```python
from build123d import *

# Parameters (mm, degrees)
BOSS_EXTRUDE1_DEPTH                = 9
BOSS_EXTRUDE2_DEPTH                = 15.4
BOSS_EXTRUDE3_DEPTH                = 9
SKETCH4_R                          = 4.5
CUT_EXTRUDE1_DEPTH                 = 5
SKETCH5_R                          = 2.5
BOSS_EXTRUDE4_DEPTH                = 26.9
SKETCH6_W                          = 16.2
SKETCH6_H                          = 1.547449217
BOSS_EXTRUDE5_DEPTH                = 3.5
EXTRUDE_THIN4_DEPTH                = 6
BOSS_EXTRUDE7_DEPTH                = 0.5
SKETCH9_W                          = 16.123667198
SKETCH9_H                          = 0.274090176
BOSS_EXTRUDE8_DEPTH                = 3.5
SKETCH10_R                         = 0.25
BOSS_EXTRUDE9_DEPTH                = 5.5
CHAMFER1_SIZE                      = 0.1
SKETCH11_R                         = 11
SKETCH11_R_2                       = 4.5
BOSS_EXTRUDE10_DEPTH               = 2.5
FILLET1_R                          = 1
CUT_EXTRUDE2_DEPTH                 = 18
FILLET2_R                          = 0.5
TAP_DRILL_FOR_M2_5X0_45_TAP2_D     = 2.05
TAP_DRILL_FOR_M2_5X0_45_TAP2_DEPTH = 5
TAP_DRILL_FOR_M2_5X0_45_TAP2_TIP   = 0.615882135


with BuildPart() as part:
    # Sketch1 → Boss-Extrude1 (new body)
    with BuildSketch(Plane.XY):
        Polygon((21, 16.5), (16.5, 21), (-16.5, 21), (-21, 16.5), (-21, -16.5), (-16.5, -21), (16.5, -21), (21, -16.5), align=None)
    extrude(amount=BOSS_EXTRUDE1_DEPTH)

    # Sketch2 → Boss-Extrude2 (add)
    with BuildSketch(Plane.XY.offset(9)):
        with BuildLine():
            Line((11, 20.9), (-11, 20.9))
            ThreePointArc((-11, 20.9), (-18.000357134, 18.000357134), (-20.9, 11))
            Line((-20.9, 11), (-20.9, -11))
            ThreePointArc((-20.9, -11), (-18.000357134, -18.000357134), (-11, -20.9))
            Line((-11, -20.9), (11, -20.9))
            ThreePointArc((11, -20.9), (18.000357134, -18.000357134), (20.9, -11))
            Line((20.9, -11), (20.9, 11))
            ThreePointArc((20.9, 11), (18.000357134, 18.000357134), (11, 20.9))
        make_face()
    extrude(amount=BOSS_EXTRUDE2_DEPTH)

    # Sketch3 → Boss-Extrude3 (add)
    with BuildSketch(Plane.XY.offset(24.4)):
        Polygon((21, -16.5), (21, 16.5), (16.5, 21), (-16.5, 21), (-21, 16.5), (-21, -16.5), (-16.5, -21), (16.5, -21), align=None)
    extrude(amount=BOSS_EXTRUDE3_DEPTH)

    # Sketch4 → Cut-Extrude1 (cut)
    with BuildSketch(Plane.XY.offset(33.4)):
        Circle(SKETCH4_R)
    extrude(amount=-CUT_EXTRUDE1_DEPTH, mode=Mode.SUBTRACT)

    # Sketch5 → Boss-Extrude4 (add)
    with BuildSketch(Plane.XY.offset(28.4)):
        Circle(SKETCH5_R)
    extrude(amount=BOSS_EXTRUDE4_DEPTH)

    # Sketch6 → Boss-Extrude5 (add)
    with BuildSketch(Plane(origin=(0, 21, 0), x_dir=(1, 0, 0), z_dir=(0, 1, 0))):
        with Locations((0, -0.773724609)):
            Rectangle(SKETCH6_W, SKETCH6_H)
    extrude(amount=BOSS_EXTRUDE5_DEPTH)

    # Sketch7 → Extrude-Thin4 (add)
    with BuildSketch(Plane(origin=(0, 21, 0), x_dir=(1, 0, 0), z_dir=(0, 1, 0))):
        Polygon((-5.1, -8.547449217), (-8.1, -8.547449217), (-8.1, -2.547449217), (8.1, -2.547449217), (8.1, -8.547449217), (5.1, -8.547449217), (5.1, -8.047449217), (7.6, -8.047449217), (7.6, -3.047449217), (-7.6, -3.047449217), (-7.6, -8.047449217), (-5.1, -8.047449217), align=None)
    extrude(amount=EXTRUDE_THIN4_DEPTH)

    # Sketch8 → Boss-Extrude7 (add)
    with BuildSketch(Plane(origin=(0, 21, 0), x_dir=(1, 0, 0), z_dir=(0, 1, 0))):
        Polygon((-5.1, -8.047449217), (-5.1, -8.547449217), (5.1, -8.547449217), (5.1, -8.047449217), (7.6, -8.047449217), (7.6, -3.047449217), (-7.6, -3.047449217), (-7.6, -8.047449217), align=None)
    extrude(amount=BOSS_EXTRUDE7_DEPTH)

    # Sketch9 → Boss-Extrude8 (add)
    with BuildSketch(Plane(origin=(0, 21, 0), x_dir=(1, 0, 0), z_dir=(0, 1, 0))):
        with Locations((0, -2.039705449)):
            Rectangle(SKETCH9_W, SKETCH9_H)
    extrude(amount=BOSS_EXTRUDE8_DEPTH)

    # Sketch10 → Boss-Extrude9 (add)
    with BuildSketch(Plane(origin=(0, 21.5, 0), x_dir=(1, 0, 0), z_dir=(0, 1, 0))):
        with Locations((-6.204552759, -5.547449217)):
            Circle(SKETCH10_R)
        with Locations((-3.704552759, -5.547449217)):
            Circle(SKETCH10_R)
        with Locations((-1.204552759, -5.547449217)):
            Circle(SKETCH10_R)
        with Locations((1.295447241, -5.547449217)):
            Circle(SKETCH10_R)
        with Locations((3.795447241, -5.547449217)):
            Circle(SKETCH10_R)
        with Locations((6.295447241, -5.547449217)):
            Circle(SKETCH10_R)
    extrude(amount=BOSS_EXTRUDE9_DEPTH)

    # Chamfer1
    chamfer1_edges = [part.edges().sort_by_distance(p)[0] for p in [
        (-6.454552759, 27, 5.547449217),
        (-3.954552759, 27, 5.547449217),
        (-1.454552759, 27, 5.547449217),
        (1.045447241, 27, 5.547449217),
        (3.545447241, 27, 5.547449217),
        (6.045447241, 27, 5.547449217),
    ]]
    chamfer(chamfer1_edges, length=CHAMFER1_SIZE)

    # Sketch11 → Boss-Extrude10 (add)
    with BuildSketch(Plane.XY.offset(33.4)):
        Circle(SKETCH11_R)
        Circle(SKETCH11_R_2, mode=Mode.SUBTRACT)
    extrude(amount=BOSS_EXTRUDE10_DEPTH)

    # Fillet1
    fillet1_edges = [part.edges().sort_by_distance(p)[0] for p in [
        (-11, 0, 33.4),
    ]]
    fillet(fillet1_edges, radius=FILLET1_R)

    # Sketch12 → Cut-Extrude2 (cut)
    with BuildSketch(Plane.XY.offset(55.3)):
        with BuildLine():
            Line((2, 1.5), (-2, 1.5))
            ThreePointArc((-2, 1.5), (0, 2.5), (2, 1.5))
        make_face()
    extrude(amount=-CUT_EXTRUDE2_DEPTH, mode=Mode.SUBTRACT)

    # Fillet2
    fillet2_edges = [part.edges().sort_by_distance(p)[0] for p in [
        (-0.790569415, -2.371708245, 55.3),
    ]]
    fillet(fillet2_edges, radius=FILLET2_R)

    # Tap Drill for M2.5x0.45 Tap2
    with Locations(Plane.XY.offset(33.4)):
        with Locations((15.5, 16.5), (15.5, -16.5), (-15.5, -16.5), (-15.5, 16.5)):
            Hole(TAP_DRILL_FOR_M2_5X0_45_TAP2_D / 2, depth=TAP_DRILL_FOR_M2_5X0_45_TAP2_DEPTH)
            with Locations((0, 0, -(TAP_DRILL_FOR_M2_5X0_45_TAP2_DEPTH + TAP_DRILL_FOR_M2_5X0_45_TAP2_TIP / 2))):  # 118° drill point
                Cone(0, TAP_DRILL_FOR_M2_5X0_45_TAP2_D / 2, TAP_DRILL_FOR_M2_5X0_45_TAP2_TIP, mode=Mode.SUBTRACT)


solid = part.part
```
Geometry: final body of the model. Coordinates: model frame, mm. A direction names the side the tool comes from. Give positions to 0.01 mm unless a question says otherwise; leave off trailing zeros. Order: outer loops, then holes, each group sorted by start corner. A loop starts at its lowest first (then second) coordinate and runs counter-clockwise, first axis right, second up. Notation, with made-up numbers: M 81.25,25 L 130.25,25 A29 cw 130.25,64 Z; hole C 64,78 d2. An arc over 180 degrees is marked long. Answer as CSV lines item,"result". Start each with the question number.
1) First-contact query: P1, Ø7.5, axis at x = -3, z = 14, coming from the -Y side; P2, Ø6.5, axis at x = 0.5, y = 25.5, coming from the +Z side; P3, Ø2.5, axis at y = 24, z = 5.5, coming from the +X side. Flat tips, straight axial feed; report the tip coordinate or a pass-through.
2) Mould query, pull axis X, two halves, no side actions, for faces 1 (the flat face through (2, -2, 28.4)), 2 (the flat face through (8.1, 24, 6)), 3 (the flat face through (0, 23, 2.177)). Classes: +X half, -X half, draft (parallel to the pull), parting line (faces both ways), or undercut.
3) Line query: line 1 (Y direction, x = -15.5, z = 32.35) (3 decimals); line 2 (Y direction, x = 0, z = 30.5); line 3 (X direction, y = 16.5, z = 32) (3 decimals). Output: solid intervals per line, ascending. Write a range as from..to.
4) Cut plane C-C (x = -13). Output: boundary loops of the cut face in (y, z).
5) Cut plane B-B (z = 21.5). Output: boundary loops of the cut face in (x, y).
6) Cut plane D-D (z = 46.5). Output: boundary loops of the cut face in (x, y).
7) Cut plane A-A (y = 0). Output: boundary loops of the cut face in (x, z), then the cut area to 3 significant figures.
8) Set-up query: faces 4 (the flat face through (-8.1, 24, 6)), 5 (the flat face through (8.1, 23, 1)), 6 (the flat face through (7.6, 24, 6)), 7 (the cylindrical face through (15.633, 17.516, 30.865)). Return all of +Z, -Z, +X, -X, +Y, -Y with unobstructed straight access to the full face (end or side cutting, diameter ignored); none if empty.
Findings below:
1,P1,"stops at y = -20.9"
1,P2,"stops at z = 5.8"
1,P3,"stops at x = 8.1"
2,face 1,"undercut"
2,face 2,"+X half"
2,face 3,"draft"
3,line 1,"y = -21..-17.525, -15.475..15.475, 17.525..21"
3,line 2,"y = -21..-4.5, -2.5..2.5, 4.5..21"
3,line 3,"x = -21..-16.525, -14.475..14.475, 16.525..21"
4,outline,"M -21,0 L 21,0 L 21,9 L 20.7,9 L 20.7,24.4 L 21,24.4 L 21,33.4 L -21,33.4 L -21,24.4 L -20.7,24.4 L -20.7,9 L -21,9 Z"
5,outline,"M -20.9,-11 A9.9 ccw -11,-20.9 L 11,-20.9 A9.9 ccw 20.9,-11 L 20.9,11 A9.9 ccw 11,20.9 L -11,20.9 A9.9 ccw -20.9,11 Z"
6,outline,"M -2,1.5 A2.5 ccw long 2,1.5 Z"
7,outline,"M -21,0 L 21,0 L 21,9 L 20.9,9 L 20.9,24.4 L 21,24.4 L 21,33.4 L 12,33.4 A1 cw 11,34.4 L 11,35.9 L 4.5,35.9 L 4.5,28.4 L 2.5,28.4 L 2.5,54.8 A0.5 ccw 2,55.3 L -2,55.3 A0.5 ccw -2.5,54.8 L -2.5,28.4 L -4.5,28.4 L -4.5,35.9 L -11,35.9 L -11,34.4 A1 cw -12,33.4 L -21,33.4 L -21,24.4 L -20.9,24.4 L -20.9,9 L -21,9 Z"
7,area,"1,520 mm²"
8,face 4,"+Z, -Z, -X, +Y"
8,face 5,"+Z, -Z, +X, +Y"
8,face 6,"+Y"
8,face 7,"+Z"
